The figure shows three views and two pictorial views of one solid part (mm, origin at its lowest corner). Answer the questions. A direction names the side the tool comes from. Round coordinates to 2 decimals unless told otherwise and drop trailing zeros. Order: outer loops, then holes, each group sorted by start corner. A loop starts at its lowest first (then second) coordinate and runs counter-clockwise, first axis right, second up. Notation, with made-up numbers: (76.5, 53) - (135.5, 53) arc R20 cw to (135.5, 65) - close; hole circle Ø10 at (73.5, 88.5). An arc over 180 degrees is marked (long way). One line per question, with ' | ' between items. Start each with the question number.
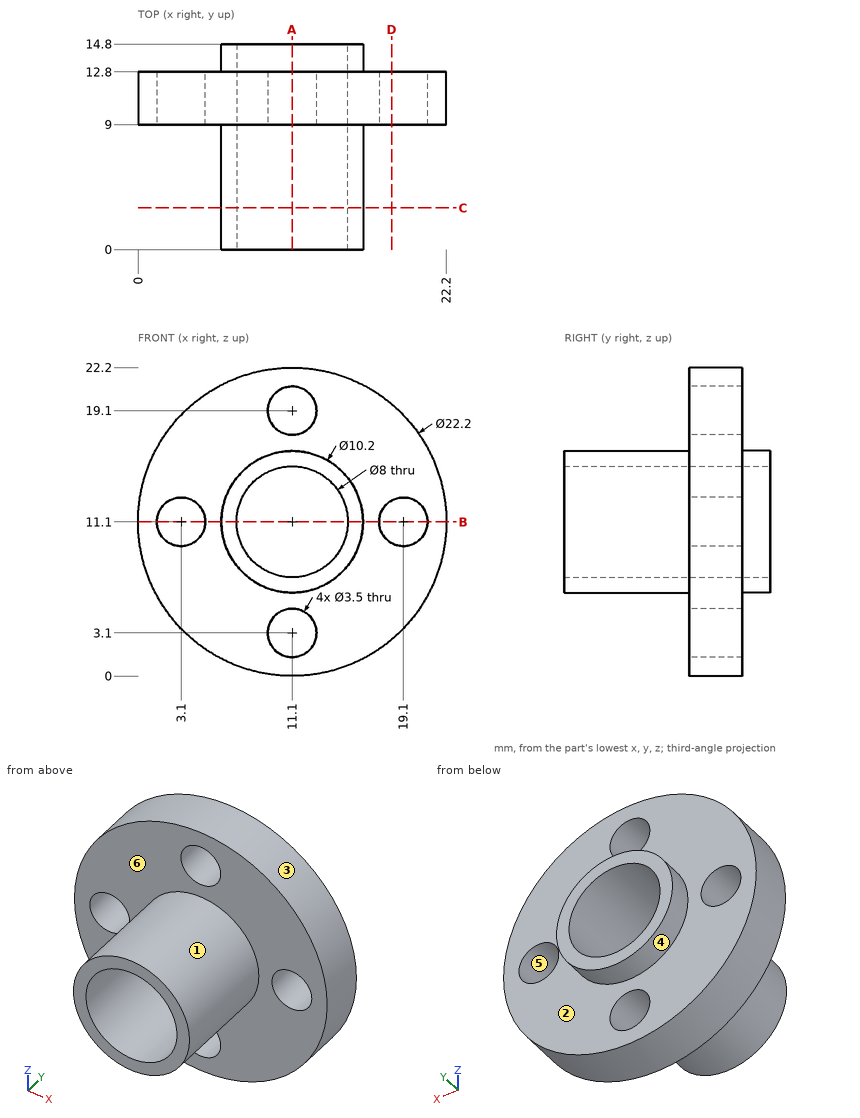
1) Section B-B on z = 11.1 is taken. Give the vertices of the cut face in (x, y).
2) Section C-C on y = 3 is taken. Give the vertices of the cut face in (x, z), and give its area (3 significant figures).
3) Determine the mould class of the marked faces 4, 5 and 6 for opening direction Z: released by +Z, released by -Z, zero draft, split by the parting line, or undercut.
4) Section D-D on x = 18.25 is taken. Give the vertices of the cut face in (y, z).
5) Flat-ended cylindrical pins translate along their axes: pin 1 (4 mm diameter, centred on x = 15.5, y = 7.5, fed in from -Z); pin 2 (2 mm diameter, centred on x = 3.1, z = 11.1, fed in from +Y); pin 3 (2 mm diameter, centred on y = 10.5, z = 19, fed in from +X); pin 4 (5 mm diameter, centred on y = 12.5, z = 10, fed in from +X). Find the tip coordinate at first contact, or state that the pin passes through.
6) For the marked faces 1, 2 and 3, determine the directions among +Z, -Z, +X, -X, +Y, -Y from which every point of the face is accessible in a straight line to the end or side of a thin tool.
7) Straight lines are drawn through the part: line 1 (X direction, y = 9.5, z = 11); line 2 (Z direction, x = 11.5, y = 9.5); line 3 (Z direction, x = 11.1, y = 8.75). For each, find the intervals that lie inside material, in ascending order.
8) Section A-A on x = 11.1 is taken. Give the vertices of the cut face in (y, z).
Recorded:
1) outline: (0, 9) - (1.35, 9) - (1.35, 12.8) - (0, 12.8) - close; (4.85, 9) - (6, 9) - (6, 0) - (7.1, 0) - (7.1, 14.8) - (6, 14.8) - (6, 12.8) - (4.85, 12.8) - close; (15.1, 0) - (16.2, 0) - (16.2, 9) - (17.35, 9) - (17.35, 12.8) - (16.2, 12.8) - (16.2, 14.8) - (15.1, 14.8) - close; (20.85, 9) - (22.2, 9) - (22.2, 12.8) - (20.85, 12.8) - close
2) outline: circle Ø10.2 at (11.1, 11.1); hole circle Ø8 at (11.1, 11.1) | area: 31.4 mm²
3) face 4: split by the parting line | face 5: undercut | face 6: zero draft
4) outline: (9, 2.61) - (12.8, 2.61) - (12.8, 9.57) - (9, 9.57) - close; (9, 12.63) - (12.8, 12.63) - (12.8, 19.59) - (9, 19.59) - close
5) pin 1: stops at z = 0.44 | pin 2: passes through | pin 3: stops at x = 19.79 | pin 4: stops at x = 22.2
6) face 1: -Y | face 2: +Y | face 3: +Y, -Y
7) line 1: x = 0 to 1.35, 4.85 to 7.1, 15.1 to 17.35, 20.85 to 22.2 | line 2: z = 0.01 to 1.4, 4.8 to 7.12, 15.08 to 17.4, 20.8 to 22.19 | line 3: z = 6 to 7.1, 15.1 to 16.2
8) outline: (0, 6) - (9, 6) - (9, 4.85) - (12.8, 4.85) - (12.8, 6) - (14.8, 6) - (14.8, 7.1) - (0, 7.1) - close; (0, 15.1) - (14.8, 15.1) - (14.8, 16.2) - (12.8, 16.2) - (12.8, 17.35) - (9, 17.35) - (9, 16.2) - (0, 16.2) - close; (9, 0) - (12.8, 0) - (12.8, 1.35) - (9, 1.35) - close; (9, 20.85) - (12.8, 20.85) - (12.8, 22.2) - (9, 22.2) - close
